```python
from build123d import *

# Parameters (mm, degrees)
SKETCH1_W           = 25
SKETCH1_H           = 15
SKETCH1_R           = 1
BOSS_EXTRUDE1_DEPTH = 2
FILLET5_R           = 1
SKETCH2_W           = 25
SKETCH2_H           = 15
BOSS_EXTRUDE2_DEPTH = 2
FILLET6_R           = 1
FILLET7_R           = 1
SKETCH3_R           = 1
CUT_EXTRUDE1_DEPTH  = 32


with BuildPart() as part:
    # Sketch1 → Boss-Extrude1 (new body)
    with BuildSketch(Plane.XY):
        with Locations((-12.5, -7.5)):
            Rectangle(SKETCH1_W, SKETCH1_H)
        with Locations((-23.519315542, -13.423068426)):
            Circle(SKETCH1_R, mode=Mode.SUBTRACT)
        with Locations((-1.508210611, -13.423068426)):
            Circle(SKETCH1_R, mode=Mode.SUBTRACT)
    extrude(amount=BOSS_EXTRUDE1_DEPTH)

    # Fillet5
    fillet5_edges = [part.edges().sort_by_distance(p)[0] for p in [
        (0, -15, 1),
        (-25, -15, 1),
    ]]
    fillet(fillet5_edges, radius=FILLET5_R)

    # Sketch2 → Boss-Extrude2 (add)
    with BuildSketch(Plane(origin=(0, 0, 0), x_dir=(1, 0, 0), z_dir=(0, 1, 0))):
        with Locations((-12.5, 5.5)):
            Rectangle(SKETCH2_W, SKETCH2_H)
    extrude(amount=BOSS_EXTRUDE2_DEPTH)

    # Fillet6
    fillet6_edges = [part.edges().sort_by_distance(p)[0] for p in [
        (-25, 1, -13),
    ]]
    fillet(fillet6_edges, radius=FILLET6_R)

    # Fillet7
    fillet7_edges = [part.edges().sort_by_distance(p)[0] for p in [
        (0, 1, -13),
    ]]
    fillet(fillet7_edges, radius=FILLET7_R)

    # Sketch3 → Cut-Extrude1 (cut)
    with BuildSketch(Plane(origin=(0, 2, 0), x_dir=(1, 0, 0), z_dir=(0, 1, 0))):
        with Locations((-12.5, 10.148186861)):
            Circle(SKETCH3_R)
    extrude(amount=-CUT_EXTRUDE1_DEPTH, mode=Mode.SUBTRACT)


solid = part.part
```
CAD build for the part. Positions are in the model's coordinates, mm. A direction names the side the tool comes from. Round coordinates to 2 decimals unless told otherwise and drop trailing zeros. Loops run counter-clockwise (first coordinate to the right, second up) from the corner with the lowest first, then second, coordinate; pieces in that order, holes last. Notation, with made-up numbers: (45.25, 54.5) - (55.25, 54.5) arc R32 ccw to (55.25, 88.5) - close; hole circle Ø9 at (-34.5, -9.5). An arc over 180 degrees is marked (long way). Return JSON: item names as keys, results as strings. Group by question number.
Q1. Drill centre line: line 1 along Y through (x, z) = (-19.75, -9.25). Where is it in solid material? Low to high. Write a range as [from, to].
Q2. Band-saw the part on C-C on z = 0.5. Give the cut face in (x, y).
Q3. Two-plate mould, pull along Y, no slides. Class faces 3 (the face through (-1.05, -14.31, 0.99)), 4 (the face through (-13, 1, -13)), 5 (the face through (-13, 0, -7)): +Y half, -Y half, draft (parallel to the pull), parting line (faces both ways), or undercut.
Q4. Flat gauge pins, fed straight in: pin 1 Ø6 at (x, z) = (-10.5, -8) entering from -Y; pin 2 Ø2 at (x, y) = (-14.5, -13) entering from -Z. Where does each tip first touch, or does it go through?
Q5. Tool access for faces 1 (the face through (-13, -7, 0)), 2 (the face through (-24.313, -14.032, 0.986)): list every direction of +Z, -Z, +X, -X, +Y, -Y with a clear straight run to the whole face (end or side of a thin tool).
Q6. Band-saw the part on D-D on x = -15.25. Give the cut face in (y, z).
Q7. Band-saw the part on A-A on x = -12.5. Give the cut face in (y, z).
Q8. Band-saw the part on B-B on z = -10.5. Give the cut face in (x, y).
Solutions:
{
 "1": {"line 1": "y = [0, 2]"},
 "2": {"outline": "(-25, -14) arc R1 ccw to (-24, -15) - (-1, -15) arc R1 ccw to (0, -14) - (0, 2) - (-25, 2) - close; hole circle Ø2 at (-23.52, -13.42); hole circle Ø2 at (-1.51, -13.42)"},
 "3": {"face 3": "undercut", "face 4": "draft", "face 5": "-Y half"},
 "4": {"pin 1": "stops at y = 0", "pin 2": "stops at z = 0"},
 "5": {"face 1": "-Z, +X, -X, -Y", "face 2": "+Z, -Z"},
 "6": {"outline": "(-15, 0) - (0, 0) - (0, -13) - (2, -13) - (2, 2) - (-15, 2) - close"},
 "7": {"outline": "(-15, 0) - (0, 0) - (0, -9.15) - (2, -9.15) - (2, 2) - (-15, 2) - close; (0, -13) - (2, -13) - (2, -11.15) - (0, -11.15) - close"},
 "8": {"outline": "(-25, 0) - (-13.44, 0) - (-13.44, 2) - (-25, 2) - close; (-11.56, 0) - (0, 0) - (0, 2) - (-11.56, 2) - close"}
}
